Design review of the part shown in the three views and the two pictorial views. Dimensions are in mm from the part's minimum x, y and z. Coordinates: 2 decimals unless noted, no trailing zeros. Loops run counter-clockwise (first coordinate to the right, second up) from the corner with the lowest first, then second, coordinate; pieces in that order, holes last. Notation, with made-up numbers: (-4, -25.5) -> (17, -25.5) arc R14 cw to (17, -16.5) -> close; hole circle Ø1 at (-16, 18). An arc over 180 degrees is marked (long way). Answer in a Markdown table with one row per item.
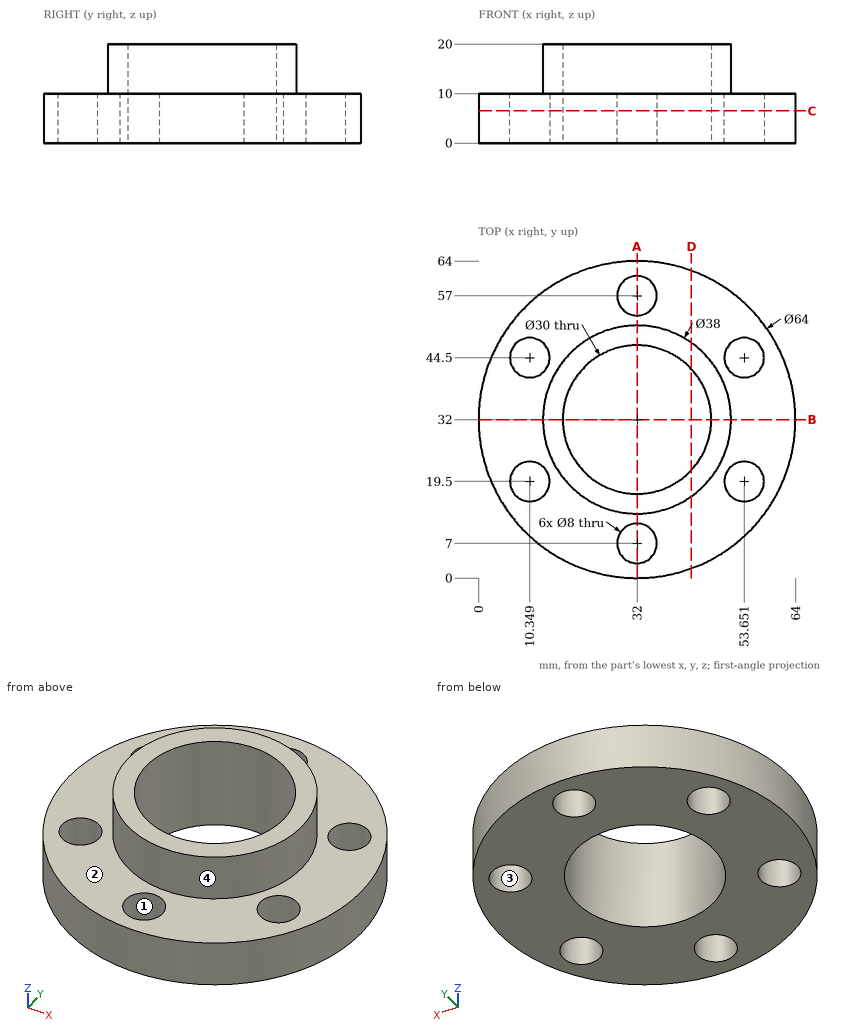
Item 1: Take a section at B-B, the plane y = 32. State the section outline as (x, z) points.
Worked answers:
| item | result |
|---|---|
| outline | (0, 0) -> (17, 0) -> (17, 20) -> (13, 20) -> (13, 10) -> (0, 10) -> close; (47, 0) -> (64, 0) -> (64, 10) -> (51, 10) -> (51, 20) -> (47, 20) -> close |
Item 2: Take a section at C-C, the plane z = 6.5. State the section outline as (x, y) points, and give its area (3 significant figures).
Worked answers:
| item | result |
|---|---|
| outline | circle Ø64 at (32, 32); hole circle Ø8 at (10.35, 19.5); hole circle Ø8 at (10.35, 44.5); hole circle Ø30 at (32, 32); hole circle Ø8 at (32, 7); hole circle Ø8 at (32, 57); hole circle Ø8 at (53.65, 19.5); hole circle Ø8 at (53.65, 44.5) |
| area | 2,210 mm² |
Item 3: Insertion check: pin 1 (3 mm diameter, centred on x = 11.5, z = 10, fed in from -Y); pin 2 (6 mm diameter, centred on x = 30.5, z = 7.5, fed in from +Y); pin 3 (10.5 mm diameter, centred on x = 10.35, y = 19.5, fed in from +Z). Each pin has a flat end and moves straight along its axis. Give the tip position at first contact, or say it passes through.
Worked answers:
| item | result |
|---|---|
| pin 1 | y = 6.25 |
| pin 2 | y = 64 |
| pin 3 | z = 10 |
Item 4: The part is to be moulded in two halves that separate along X. For the marked faces 1, 2, 3 and 4, say which applies: +X half, -X half, draft (parallel to the pull), parting line (faces both ways), or undercut.
Worked answers:
| item | result |
|---|---|
| face 1 | undercut |
| face 2 | draft |
| face 3 | undercut |
| face 4 | parting line |
Item 5: For L1, parallel to Y at x = 32, z = 3; L2, parallel to X at y = 31.5, z = 13.5; L3, parallel to Y at x = 32, z = 17, list the stretches that pass through material, from the lowest coordinate up.
Worked answers:
| item | result |
|---|---|
| L1 | 0 to 3, 11 to 17, 47 to 53, 61 to 64 |
| L2 | 13.01 to 17.01, 46.99 to 50.99 |
| L3 | 13 to 17, 47 to 51 |
Item 6: Take a section at A-A, the plane x = 32. State the section outline as (y, z) points.
Worked answers:
| item | result |
|---|---|
| outline | (0, 0) -> (3, 0) -> (3, 10) -> (0, 10) -> close; (11, 0) -> (17, 0) -> (17, 20) -> (13, 20) -> (13, 10) -> (11, 10) -> close; (47, 0) -> (53, 0) -> (53, 10) -> (51, 10) -> (51, 20) -> (47, 20) -> close; (61, 0) -> (64, 0) -> (64, 10) -> (61, 10) -> close |
Item 7: Take a section at D-D, the plane x = 43. State the section outline as (y, z) points, and give its area (3 significant figures).
Worked answers:
| item | result |
|---|---|
| outline | (1.95, 0) -> (21.8, 0) -> (21.8, 20) -> (16.51, 20) -> (16.51, 10) -> (1.95, 10) -> close; (42.2, 0) -> (62.05, 0) -> (62.05, 10) -> (47.49, 10) -> (47.49, 20) -> (42.2, 20) -> close |
| area | 503 mm² |
